Design review of the part shown in the three views and the two pictorial views. Dimensions are in mm from the part's minimum x, y and z. Round coordinates to 2 decimals unless told otherwise and drop trailing zeros. Write each loop counter-clockwise with the first axis right and the second up, starting at its lowest first coordinate (ties: lowest second). Pieces come first, ordered by that corner, then holes. Notation, with made-up numbers: (-18, -26.75) -> (34, -26.75) arc R23 ccw to (34, 7.25) -> close; hole circle Ø7 at (87, 50.25). An arc over 180 degrees is marked (long way). One line per question, with ' | ' between items. Start each with the question number.
1) Consider section B-B (z = 3.9). Give the boundary of the cut face in (x, y), then the cut area to 3 significant figures.
2) Insertion check: pin 1 Ø3 at (x, y) = (7.5, 7.5) entering from -Z. The pin has a flat end and moves straight along its axis. Give the tip position at first contact, or say it passes through.
3) Mouldability with a two-part tool opening along X and no side actions: class the marked faces 1, 2, 3 and 4 as +X half, -X half, draft (parallel to the pull), parting line (faces both ways), or undercut.
4) Consider section A-A (x = 57.5). Give the boundary of the cut face in (y, z).
5) For probe 1 along Y at (x, z) = (7.5, 1.9); probe 2 along Y at (x, z) = (82.5, 2.25); probe 3 along X at (y, z) = (9, 5.05), list the stretches that pass through material, from the lowest coordinate up.
6) Consider section C-C (y = 1.5). Give the boundary of the cut face in (x, z), then the cut area to 3 significant figures.
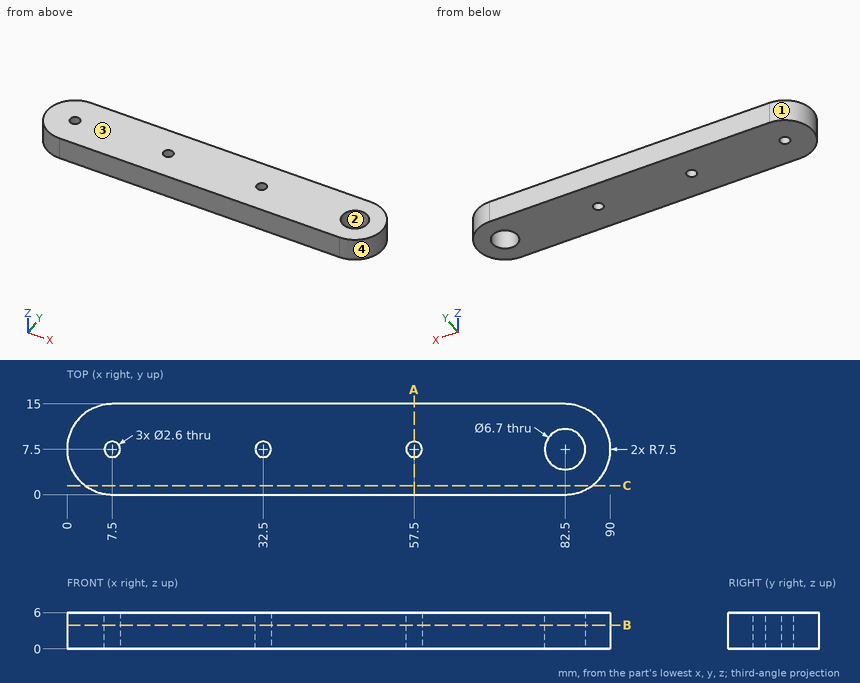
From the geometry:
1) outline: (7.5, 0) -> (82.5, 0) arc R7.5 ccw to (82.5, 15) -> (7.5, 15) arc R7.5 ccw to start; hole circle Ø2.6 at (7.5, 7.5); hole circle Ø2.6 at (32.5, 7.5); hole circle Ø2.6 at (57.5, 7.5); hole circle Ø6.7 at (82.5, 7.5) | area: 1,250 mm2
2) pin 1: stops at z = 0
3) face 1: -X half | face 2: undercut | face 3: draft | face 4: +X half
4) outline: (0, 0) -> (6.2, 0) -> (6.2, 6) -> (0, 6) -> close; (8.8, 0) -> (15, 0) -> (15, 6) -> (8.8, 6) -> close
5) probe 1: y = 0 to 6.2, 8.8 to 15 | probe 2: y = 0 to 4.15, 10.85 to 15 | probe 3: x = 0.15 to 79.5, 85.5 to 89.85
6) outline: (3, 0) -> (87, 0) -> (87, 6) -> (3, 6) -> close | area: 504 mm2
